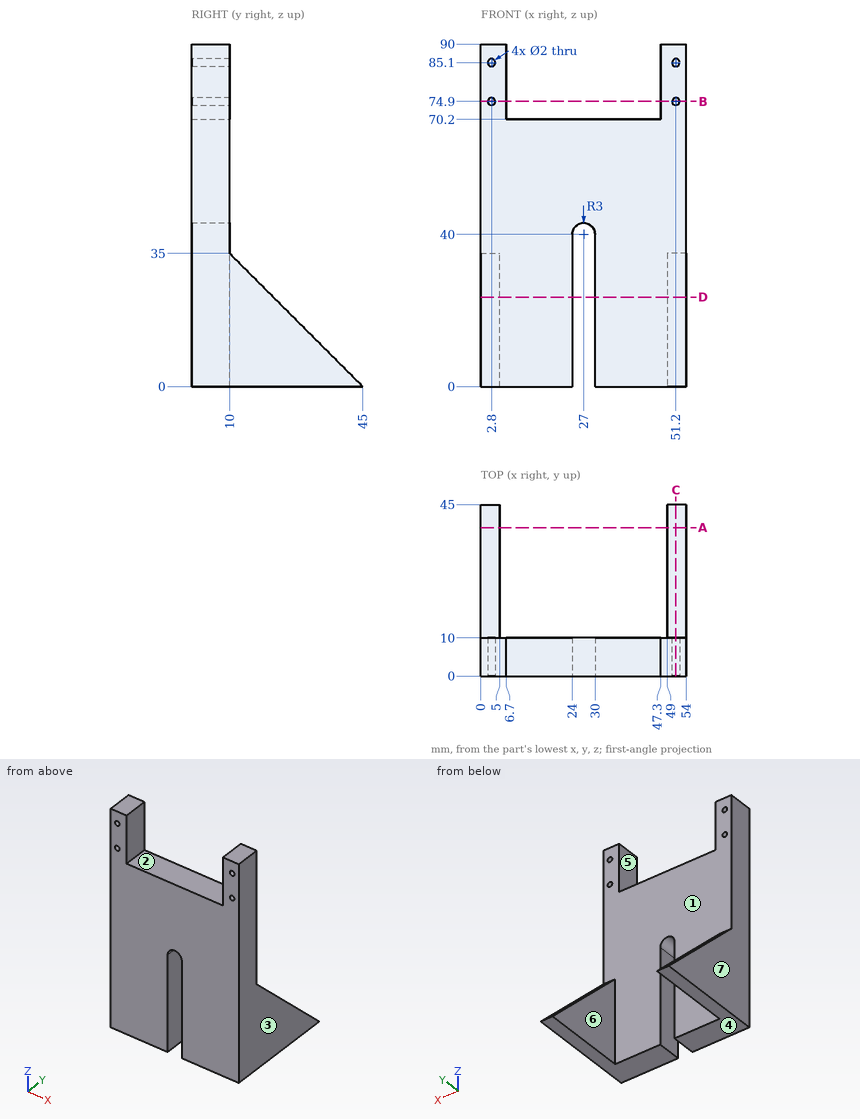
Could you check a few things on this drawing? It's one solid part, dimensions in mm from its lowest x, y, z. A direction names the side the tool comes from. Give positions to 0.01 mm unless a question says otherwise; leave off trailing zeros. Order: outer loops, then holes, each group sorted by start corner. A loop starts at its lowest first (then second) coordinate and runs counter-clockwise, first axis right, second up. Notation, with made-up numbers: (65, -6) - (86, -6) arc R28 ccw to (86, 26) - close; hole circle Ø10 at (64, 20). An arc over 180 degrees is marked (long way). Return JSON: item names as keys, results as strings. Group by question number.
Q1. Suppose I cut it at A-A, the plane y = 39. Please give me the cut outline in (x, z).
Q2. Thinking about a two-plate mould opening in X: for the marked faces 1, 2, 3 and 4, which applies, pulls with the +X half, pulls with the -X half, needs draft (parallel to the pull), parting line crosses it, or undercut?
Q3. Which directions (+Z, -Z, +X, -X, +Y, -Y) give clear straight access to the entire face, cutting with the end or side of a thin tool? Please do the marked faces 5, 6 and 7.
Q4. Please list where these lines run through material, in increasing order: line 1 along X through (y, z) = (3.5, 85.1); line 2 along Z through (x, y) = (51, 7); line 3 along Y through (x, z) = (7, 59.5). Write a range as [from, to].
Q5. Suppose I cut it at B-B, the plane z = 74.9. Please give me the cut outline in (x, y).
Q6. Will these pins go through, and if not, where does the flat tip stop? pin 1 Ø8 at (x, y) = (12, 28.5) entering from -Z; pin 2 Ø5 at (x, y) = (35, 6.5) entering from +Z.
Q7. Suppose I cut it at D-D, the plane z = 23.5. Please give me the cut outline in (x, y), and give its area (3 significant figures).
Q8. Suppose I cut it at C-C, the plane x = 51.2. Please give me the cut outline in (y, z).
Resolved:
{
 "1": {"outline": "(0, 0) - (5, 0) - (5, 6) - (0, 6) - close; (49, 0) - (54, 0) - (54, 6) - (49, 6) - close"},
 "2": {"face 1": "undercut", "face 2": "undercut", "face 3": "pulls with the +X half", "face 4": "needs draft"},
 "3": {"face 5": "+Z, +Y, -Y", "face 6": "+Z, -Z, +Y", "face 7": "+Z, -Z, -X, +Y, -Y"},
 "4": {"line 1": "x = [0, 1.8], [3.8, 6.7], [47.3, 50.2], [52.2, 54]", "line 2": "z = [0, 73.92], [75.88, 84.12], [86.08, 90]", "line 3": "y = [0, 10]"},
 "5": {"outline": "(0, 0) - (1.8, 0) - (1.8, 10) - (0, 10) - close; (3.8, 0) - (6.7, 0) - (6.7, 10) - (3.8, 10) - close; (47.3, 0) - (50.2, 0) - (50.2, 10) - (47.3, 10) - close; (52.2, 0) - (54, 0) - (54, 10) - (52.2, 10) - close"},
 "6": {"pin 1": "passes through", "pin 2": "stops at z = 70.2"},
 "7": {"outline": "(0, 0) - (24, 0) - (24, 10) - (5, 10) - (5, 21.5) - (0, 21.5) - close; (30, 0) - (54, 0) - (54, 21.5) - (49, 21.5) - (49, 10) - (30, 10) - close", "area": "595 mm2"},
 "8": {"outline": "(0, 0) - (45, 0) - (10, 35) - (10, 73.9) - (0, 73.9) - close; (0, 75.9) - (10, 75.9) - (10, 84.1) - (0, 84.1) - close; (0, 86.1) - (10, 86.1) - (10, 90) - (0, 90) - close"}
}
